Drawing for the job (mm, zero at the part's lowest x, y, z). A direction names the side the tool comes from. Give positions to 0.01 mm unless a question says otherwise; leave off trailing zeros. Loops run counter-clockwise (first coordinate to the right, second up) from the corner with the lowest first, then second, coordinate; pieces in that order, holes last.
1) Band-saw the part on B-B on y = 73. List the corners of the cut face in (x, z).
2) Band-saw the part on A-A on x = 171.7. List the corners of the cut face in (y, z).
3) Band-saw the part on C-C on z = 7. List the corners of the cut face in (x, y), then the cut area to 3 significant figures.
4) 3-axis set-ups, long thin cutter, end or side, ignore diameter. For the marked faces 1 and 2: which of +Z, -Z, +X, -X, +Y, -Y reach the whole face in a straight line?
5) Wall check: line 1 (Y direction, x = 171.7, z = 1.3); line 2 (X direction, y = 55.5, z = 2.5); line 3 (Z direction, x = 169, y = 75.5). Give the ranges that are in metal, low to high.
6) Flat gauge pins, fed straight in: P1, Ø8, axis at y = 36, z = 11.5, coming from the -X side; P2, Ø17, axis at x = 9.5, y = 50, coming from the +Z side; P3, Ø4.5, axis at x = 171.7, y = 40.9, coming from the -Z side; P4, Ø5, axis at y = 62, z = 13.5, coming from the +X side. Where does each tip first touch, or does it go through?
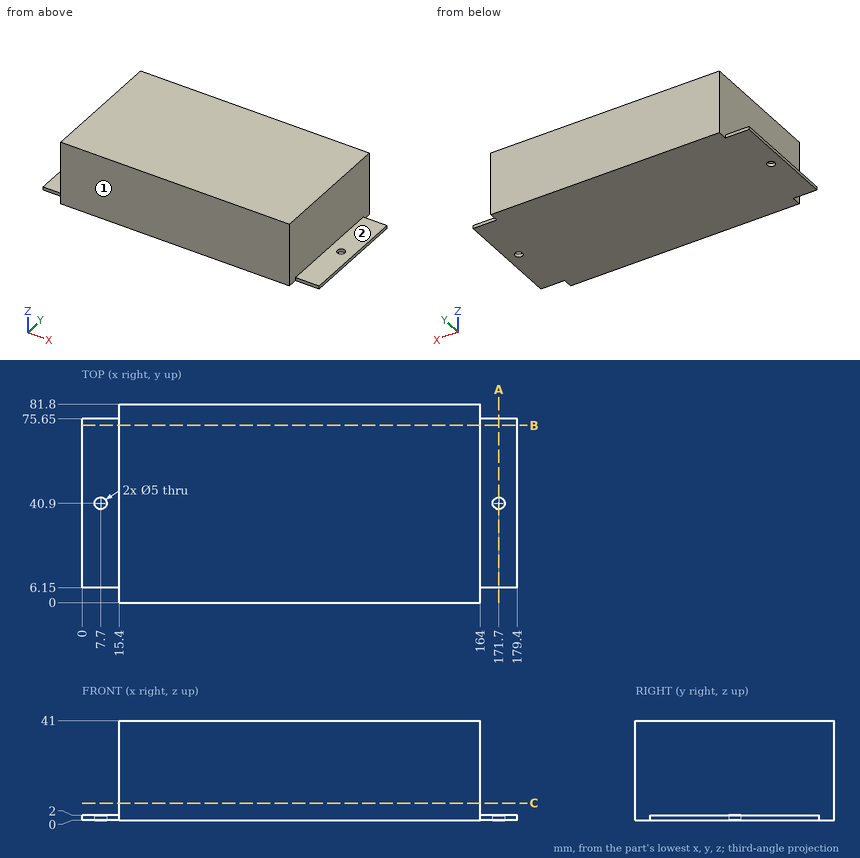
Findings below:
1. outline: (0, 0) - (179.4, 0) - (179.4, 2) - (164, 2) - (164, 41) - (15.4, 41) - (15.4, 2) - (0, 2) - close
2. outline: (6.15, 0) - (38.4, 0) - (38.4, 2) - (6.15, 2) - close; (43.4, 0) - (75.65, 0) - (75.65, 2) - (43.4, 2) - close
3. outline: (15.4, 0) - (164, 0) - (164, 81.8) - (15.4, 81.8) - close
3. area: 12,200 mm2
4. face 1: +Z, -Z, +X, -X, -Y
4. face 2: +Z, +X, +Y, -Y
5. line 1: y = 6.15 to 38.4, 43.4 to 75.65
5. line 2: x = 15.4 to 164
5. line 3: z = 0 to 2
6. P1: stops at x = 15.4
6. P2: stops at z = 41
6. P3: passes through
6. P4: stops at x = 164
